Design review of the part built by this model. Coordinates are the model's own, in mm. Round coordinates to 2 decimals unless told otherwise and drop trailing zeros. Loops run counter-clockwise (first coordinate to the right, second up) from the corner with the lowest first, then second, coordinate; pieces in that order, holes last. Notation, with made-up numbers: (39, -15) -> (65, -15) arc R27 cw to (65, 5) -> close; hole circle Ø1 at (-38, -25). An arc over 180 degrees is marked (long way). Use a Markdown table: item, result. Add a question column.
from build123d import *

# Parameters (mm, degrees)
F0_R     = 7.9375
F0_R_2   = 6.5
F1_DEPTH = 11.43
F2_R     = 0.6
F3_R     = 0.6


with BuildPart() as f1:
    # F0 (on Top) → F1 (new body)
    with BuildSketch(Plane.XY):
        Circle(F0_R)
        Circle(F0_R_2, mode=Mode.SUBTRACT)
    extrude(amount=F1_DEPTH)

    # F2
    f2_edges = [f1.edges().sort_by_distance(p)[0] for p in [
        (-6.5, 0, 0),
        (-7.9375, 0, 11.43),
        (-6.5, 0, 11.43),
    ]]
    fillet(f2_edges, radius=F2_R)

    # F3
    f3_edges = [f1.edges().sort_by_distance(p)[0] for p in [
        (-7.9375, 0, 0),
    ]]
    fillet(f3_edges, radius=F3_R)


solid = f1.part
1. Consider section A-A on x = 0. State the section outline as (y, z) points.
2. Insertion check: P1, Ø6, axis at x = 3, y = -5, coming from the +Z side; P2, Ø5, axis at y = -4.5, z = 7, coming from the -X side; P3, Ø3, axis at x = 3.5, z = 8.5, coming from the +Y side; P4, Ø3, axis at x = -6, z = 10, coming from the +Y side. Each pin has a flat end and moves straight along its axis. Give the tip position at first contact, or say it passes through.
3. Mouldability with a two-part tool opening along X and no side actions: class faces 1 (the face through (-5.158, -3.955, 5.643)), 2 (the face through (-1.72, -7.75, 5.64)) as +X half, -X half, draft (parallel to the pull), parting line (faces both ways), or undercut.
4. Consider section C-C on z = 8.25. State the section outline as (x, y) points (1 decimal).
5. To check wall thickness, follow probe 1 along X at (y, z) = (0.25, 3.5); probe 2 along Y at (x, z) = (0, 3); probe 3 along Y at (x, z) = (-3.25, 3.75). State the ranges of each line that lie inside material, in increasing order. Write a range as from..to.
Verdict:
| question | item | result |
|---|---|---|
| 1 | outline | (-7.94, 0.6) arc R0.6 ccw to (-7.34, 0) -> (-7.1, 0) arc R0.6 ccw to (-6.5, 0.6) -> (-6.5, 10.83) arc R0.6 ccw to (-7.1, 11.43) -> (-7.34, 11.43) arc R0.6 ccw to (-7.94, 10.83) -> close; (6.5, 0.6) arc R0.6 ccw to (7.1, 0) -> (7.34, 0) arc R0.6 ccw to (7.94, 0.6) -> (7.94, 10.83) arc R0.6 ccw to (7.34, 11.43) -> (7.1, 11.43) arc R0.6 ccw to (6.5, 10.83) -> close |
| 2 | P1 | stops at z = 11.43 |
| 2 | P2 | stops at x = -7.68 |
| 2 | P3 | stops at y = 7.68 |
| 2 | P4 | stops at y = 6.54 |
| 3 | face 1 | undercut |
| 3 | face 2 | parting line |
| 4 | outline | circle Ø15.9 at (0, 0); hole circle Ø13 at (0, 0) |
| 5 | probe 1 | x = -7.93..-6.5, 6.5..7.93 |
| 5 | probe 2 | y = -7.94..-6.5, 6.5..7.94 |
| 5 | probe 3 | y = -7.24..-5.63, 5.63..7.24 |
